Check sheet for the modelled part. Datum: model origin and axes. Units: mm. A direction names the side the tool comes from. Give positions to 0.01 mm unless a question says otherwise; leave off trailing zeros. Order: outer loops, then holes, each group sorted by start corner. A loop starts at its lowest first (then second) coordinate and runs counter-clockwise, first axis right, second up.
Item 1: Sectioned sample at A-A on x = 0. Record the boundary of the cut face in (y, z).
Item 2: Release check for a two-part mould opening along X. For faces 1 (the cylindrical face through (30.736, 2.218, -4.036)), 2 (the flat face through (0, 12.7, 0)), 3 (the cylindrical face through (-10.4, 7.9, 8.7)) record: released by +X, released by -X, zero draft, split by the parting line, or undercut.
Item 3: Material ranges on line 1 along X through (y, z) = (2.25, -11.5); line 2 along Z through (x, y) = (-12, 12.25); line 3 along Y through (x, z) = (-6, -3), recorded low to high.
Item 4: Access from +Z, -Z, +X, -X, +Y, -Y to the whole of each face (thin tool, end or side, straight path). Record for faces 4 (the cylindrical face through (-16.108, 8.803, -3.577)), 5 (the cylindrical face through (-2.325, 7.85, -13.357)), 6 (the cylindrical face through (-4.195, 3.131, 12.305)).
Item 5: Sectioned sample at B-B on y = 8.5. Count the separate pieces of the cut face and the enclosed holes in it, and give its area (3 significant figures).
Item 6: Gauge pin test, flat ends, axial feed: P1, Ø3, axis at x = -18.42, z = 12.93, coming from the -Y side; P2, Ø6, axis at x = 7, y = 5.5, coming from the -Z side; P3, Ø1, axis at x = 21.5, z = 10, coming from the +Y side; P4, Ø1.5, axis at x = -10.5, y = 10.5, coming from the +Z side. Record the tip position at first contact, or that the pin passes through.
from build123d import *

# Parameters (mm, degrees)
SKETCH1_R           = 31
SKETCH1_R_2         = 13
BOSS_EXTRUDE1_DEPTH = 6.35
SKETCH3_R           = 2
CUT_EXTRUDE1_DEPTH  = 45.29810944
SKETCH2_R           = 16.5
BOSS_EXTRUDE2_DEPTH = 6.35
SKETCH4_R           = 1.6
CUT_EXTRUDE2_DEPTH  = 46.643071763
SKETCH5_R           = 2
CUT_EXTRUDE3_DEPTH  = 46.643071763
CUT_EXTRUDE4_START  = -1.35
SKETCH7_R           = 31
SKETCH7_R_2         = 16.5
CUT_EXTRUDE4_DEPTH  = 1.35
FILLET1_R           = 0.5


with BuildPart() as part:
    # Sketch1 → Boss-Extrude1 (new body)
    with BuildSketch(Plane(origin=(0, 0, 0), x_dir=(1, 0, 0), z_dir=(0, 1, 0))):
        with Locations(Location((0, 0, 0), (0, 0, 270))):
            Circle(SKETCH1_R)
        with Locations(Location((0, 0, 0), (0, 0, 270))):
            Circle(SKETCH1_R_2, mode=Mode.SUBTRACT)
    extrude(amount=BOSS_EXTRUDE1_DEPTH)

    # Sketch3 → Cut-Extrude1 (cut, through all)
    with BuildSketch(Plane.XZ):
        with Locations(Location((-3.881517499, 22.162667301, 0), (0, 0, 270))):
            Circle(SKETCH3_R)
        with Locations(Location((-12.926724993, -18.416019683, 0), (0, 0, 270))):
            Circle(SKETCH3_R)
        with Locations(Location((3.881517499, -22.162667301, 0), (0, 0, 270))):
            Circle(SKETCH3_R)
        with Locations(Location((18.416019683, -12.926724993, 0), (0, 0, 270))):
            Circle(SKETCH3_R)
        with Locations(Location((22.162667301, 3.881517499, 0), (0, 0, 270))):
            Circle(SKETCH3_R)
        with Locations(Location((12.926724993, 18.416019683, 0), (0, 0, 270))):
            Circle(SKETCH3_R)
        with Locations(Location((-18.416019683, 12.926724993, 0), (0, 0, 270))):
            Circle(SKETCH3_R)
        with Locations(Location((-22.162667301, -3.881517499, 0), (0, 0, 270))):
            Circle(SKETCH3_R)
    extrude(amount=-CUT_EXTRUDE1_DEPTH, mode=Mode.SUBTRACT)

    # Sketch2 → Boss-Extrude2 (add)
    with BuildSketch(Plane(origin=(0, 6.35, 0), x_dir=(1, 0, 0), z_dir=(0, 1, 0))):
        with Locations(Location((0, 0, 0), (0, 0, 270))):
            Circle(SKETCH2_R)
    extrude(amount=BOSS_EXTRUDE2_DEPTH)

    # Sketch4 → Cut-Extrude2 (cut, through all)
    with BuildSketch(Plane(origin=(0, 12.7, 0), x_dir=(1, 0, 0), z_dir=(0, 1, 0))):
        with Locations(Location((-8.985259132, -7.953937285, 0), (0, 0, 270))):
            Circle(SKETCH4_R)
        with Locations(Location((-11.380941315, 3.804494025, 0), (0, 0, 270))):
            Circle(SKETCH4_R)
        with Locations(Location((-2.395682183, 11.75843131, 0), (0, 0, 270))):
            Circle(SKETCH4_R)
        with Locations(Location((8.985259131, 7.953937285, 0), (0, 0, 270))):
            Circle(SKETCH4_R)
        with Locations(Location((11.380941314, -3.804494026, 0), (0, 0, 270))):
            Circle(SKETCH4_R)
        with Locations(Location((2.395682183, -11.75843131, 0), (0, 0, 270))):
            Circle(SKETCH4_R)
    extrude(amount=-CUT_EXTRUDE2_DEPTH, mode=Mode.SUBTRACT)

    # Sketch5 → Cut-Extrude3 (cut, through all)
    with BuildSketch(Plane(origin=(0, 12.7, 0), x_dir=(1, 0, 0), z_dir=(0, 1, 0))):
        with Locations(Location((-2.805814344, -8.393444219, 0), (0, 0, 270))):
            Circle(SKETCH5_R)
        with Locations(Location((-5.866028748, 6.626628609, 0), (0, 0, 270))):
            Circle(SKETCH5_R)
        with Locations(Location((8.671843091, 1.76681561, 0), (0, 0, 270))):
            Circle(SKETCH5_R)
    extrude(amount=-CUT_EXTRUDE3_DEPTH, mode=Mode.SUBTRACT)

    # Sketch7 → Cut-Extrude4 (cut)
    with BuildSketch(Plane(origin=(0, 6.35, 0), x_dir=(1, 0, 0), z_dir=(0, 1, 0)).offset(CUT_EXTRUDE4_START)):
        with Locations(Location((0, 0, 0), (0, 0, 270))):
            Circle(SKETCH7_R)
        with Locations(Location((0, 0, 0), (0, 0, 270))):
            Circle(SKETCH7_R_2, mode=Mode.SUBTRACT)
    extrude(amount=CUT_EXTRUDE4_DEPTH, mode=Mode.SUBTRACT)

    # Fillet1
    fillet1_edges = [part.edges().sort_by_distance(p)[0] for p in [
        (0, 5, -16.5),
        (0, 5, -31),
        (0, 12.7, -16.5),
    ]]
    fillet(fillet1_edges, radius=FILLET1_R)


solid = part.part
Report:
1. outline: (0, -31) - (4.5, -31) arc R0.5 ccw to (5, -30.5) - (5, -17) arc R0.5 cw to (5.5, -16.5) - (12.2, -16.5) arc R0.5 ccw to (12.7, -16) - (12.7, 16) arc R0.5 ccw to (12.2, 16.5) - (5.5, 16.5) arc R0.5 cw to (5, 17) - (5, 30.5) arc R0.5 ccw to (4.5, 31) - (0, 31) - (0, 13) - (6.35, 13) - (6.35, -13) - (0, -13) - close
2. face 1: split by the parting line
2. face 2: zero draft
2. face 3: undercut
3. line 1: x = -28.79 to -6.06, 6.06 to 17.01, 19.82 to 28.79
3. line 2: z = -11.32 to -5.28, -2.33 to 11.32
3. line 3: y = 6.35 to 12.7
4. face 4: +Y
4. face 5: +Y, -Y
4. face 6: -Y
5. separate pieces: 1
5. enclosed holes: 9
5. area: 769 mm2
6. P1: passes through
6. P2: stops at z = -30.72
6. P3: stops at y = 5
6. P4: stops at z = 13.31
